```python
from build123d import *

# Parameters (mm, degrees)
BOSS_EXTRUDE1_DEPTH = 1.5
SKETCH2_R           = 3.5
SKETCH2_R_2         = 2.5
BOSS_EXTRUDE2_DEPTH = 2.2
CUT_EXTRUDE1_REACH  = 20.87
SKETCH3_R           = 1
SKETCH4_R           = 2.5
CUT_EXTRUDE2_DEPTH  = 1


with BuildPart() as part:
    # Sketch1 → Boss-Extrude1 (new body)
    with BuildSketch(Plane.XY):
        with BuildLine():
            Line((2, 7.75863865), (2, 3.304737557))
            Line((2, 3.304737557), (14.214285714, 1.988487272))
            ThreePointArc((14.214285714, 1.988487272), (16, 0), (14.214285714, -1.988487272))
            Line((14.214285714, -1.988487272), (2, -3.304737557))
            Line((2, -3.304737557), (2, -7.75863865))
            ThreePointArc((2, -7.75863865), (0, -9.75863865), (-2, -7.75863865))
            Line((-2, -7.75863865), (-2, -3.304737557))
            Line((-2, -3.304737557), (-14.214285714, -1.988487272))
            ThreePointArc((-14.214285714, -1.988487272), (-16, 0), (-14.214285714, 1.988487272))
            Line((-14.214285714, 1.988487272), (-2, 3.304737557))
            Line((-2, 3.304737557), (-2, 7.75863865))
            ThreePointArc((-2, 7.75863865), (0, 9.75863865), (2, 7.75863865))
        make_face()
    extrude(amount=BOSS_EXTRUDE1_DEPTH)

    # Sketch2 → Boss-Extrude2 (add)
    with BuildSketch(Plane.XY.offset(1.5)):
        Circle(SKETCH2_R)
        Circle(SKETCH2_R_2, mode=Mode.SUBTRACT)
    extrude(amount=BOSS_EXTRUDE2_DEPTH)

    # Sketch3 → Cut-Extrude1 (cut, up to next)
    with BuildSketch(Plane.XY.offset(1.5), mode=Mode.PRIVATE) as cut_extrude1_sk1:
        Circle(SKETCH3_R)
    cut_extrude1_tool1 = extrude(cut_extrude1_sk1.sketch, amount=-CUT_EXTRUDE1_REACH, mode=Mode.PRIVATE) & part.part
    add(cut_extrude1_tool1.solids().sort_by_distance((0, 0, 1.5))[0], mode=Mode.SUBTRACT)

    # Sketch4 → Cut-Extrude2 (cut)
    with BuildSketch(Plane(origin=(0, 0, 0), x_dir=(-1, 0, 0), z_dir=(0, 0, -1))):
        with Locations(Location((0, 0, 0), (0, 0, 180))):
            Circle(SKETCH4_R)
    extrude(amount=-CUT_EXTRUDE2_DEPTH, mode=Mode.SUBTRACT)


solid = part.part
```
CAD build for the part. Positions are in the model's coordinates, mm. A direction names the side the tool comes from. Coordinates: 2 decimals unless noted, no trailing zeros. Order: outer loops, then holes, each group sorted by start corner. A loop starts at its lowest first (then second) coordinate and runs counter-clockwise, first axis right, second up. Notation, with made-up numbers: M -18,-8.5 L -11,-8.5 A19 cw -11,24.5 Z; hole C 29,31 d5. An arc over 180 degrees is marked long. Write each question's results on one line, items separated by ' | '. Start each with the question number.
Q1. Which spindle directions (+Z, -Z, +X, -X, +Y, -Y) get a long thin tool onto all of the face, cutting with end or side? Do faces 4 (the flat face through (2, -6, 1)), 5 (the flat face through (2, 6, 1)), 6 (the flat face through (-2, -6, 1)), 7 (the flat face through (0, -4, 1.5)), 8 (the cylindrical face through (-2.5, -0.1, 0.5)). Say none if no direction does.
Q2. Cut at C-C (y = 0). List the corners of the cut face in (x, z).
Q3. Drill centre lines: probe 1 along Y at (x, z) = (0, 1.2); probe 2 along Y at (x, z) = (0, 0.65); probe 3 along Z at (x, y) = (-6, -2.75). Where is each one in solid material? Low to high. Write a range as from..to.
Q4. Cut at D-D (y = -5.25). List the corners of the cut face in (x, z), then the cut area to 3 significant figures.
Q5. Cut at A-A (x = 0). List the corners of the cut face in (y, z), then the cut area to 3 significant figures.
Q6. Flat gauge pins, fed straight in: P1, Ø5, axis at x = 6.5, y = 2, coming from the +Z side; P2, Ø1.6, axis at y = -4.5, z = 1, coming from the +X side; P3, Ø2.5, axis at x = 1, y = -1, coming from the +Z side; P4, Ø1.6, axis at y = -6, z = 1, coming from the -X side. Where does each tip first touch, or does it go through?
Q7. Pull direction X, two halves, no side cores. Call faces 1 (the cylindrical face through (-0.217, -0.976, 1.254)), 2 (the flat face through (2.4, -1.4, 0)), 3 (the flat face through (8.193, -2.637, 0.74)): +X half, -X half, draft (parallel to the pull), parting line (faces both ways), or undercut.
Q8. Cut at B-B (z = 0.4). List the corners of the cut face in (x, y).
Found:
1) face 4: +Z, -Z, +X, -Y | face 5: +Z, -Z, +X, +Y | face 6: +Z, -Z, -X, -Y | face 7: +Z | face 8: -Z
2) outline: M -16,0 L -2.5,0 L -2.5,1 L -1,1 L -1,1.5 L -2.5,1.5 L -2.5,3.7 L -3.5,3.7 L -3.5,1.5 L -16,1.5 Z; M 1,1 L 2.5,1 L 2.5,0 L 16,0 L 16,1.5 L 3.5,1.5 L 3.5,3.7 L 2.5,3.7 L 2.5,1.5 L 1,1.5 Z
3) probe 1: -9.76..-1, 1..9.76 | probe 2: -9.76..-2.5, 2.5..9.76 | probe 3: 0..1.5
4) outline: M -2,0 L 2,0 L 2,1.5 L -2,1.5 Z | area: 6.00 mm²
5) outline: M -9.76,0 L -2.5,0 L -2.5,1 L -1,1 L -1,1.5 L -2.5,1.5 L -2.5,3.7 L -3.5,3.7 L -3.5,1.5 L -9.76,1.5 Z; M 1,1 L 2.5,1 L 2.5,0 L 9.76,0 L 9.76,1.5 L 3.5,1.5 L 3.5,3.7 L 2.5,3.7 L 2.5,1.5 L 1,1.5 Z | area: 27.7 mm²
6) P1: z = 1.5 | P2: x = 2 | P3: z = 3.7 | P4: x = -2
7) face 1: undercut | face 2: draft | face 3: +X half
8) outline: M -14.21,-1.99 L -2,-3.3 L -2,-7.76 A2 ccw 2,-7.76 L 2,-3.3 L 14.21,-1.99 A2 ccw 14.21,1.99 L 2,3.3 L 2,7.76 A2 ccw -2,7.76 L -2,3.3 L -14.21,1.99 A2 ccw Z; hole C 0,0 d5
